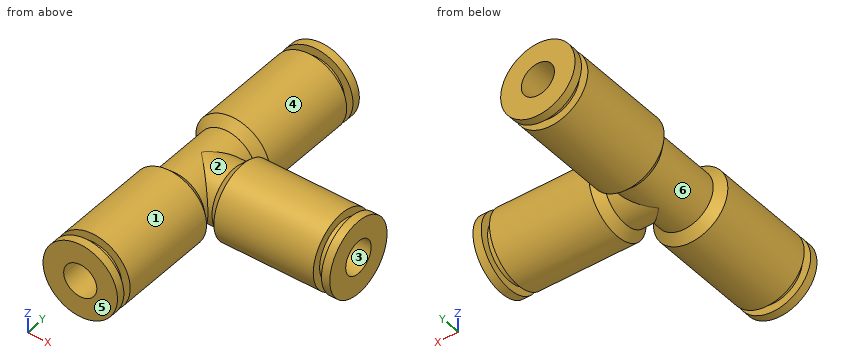
```python
from build123d import *
from build123d.topology import SkipClean

# Parameters (mm, degrees)
PATTERN_CIRCULAR_1_COUNT = 3
PATTERN_CIRCULAR_1_ANGLE = 180


with BuildPart() as part:
    # Эскиз1 one side → Повернуть1 (revolve)
    with BuildSketch(Plane.XY, mode=Mode.PRIVATE) as revolve_1_sk:
        with BuildLine():
            Line((0, -3.5), (0, -2))
            ThreePointArc((0, -2), (-1.414213562, -1.414213562), (-2, 0))
            Line((-2, 0), (-2, 6))
            Line((-2, 6), (-2, 19))
            Line((-2, 19), (-4.5, 19))
            Line((-4.5, 19), (-4.5, 18))
            Line((-4.5, 18), (-3.5, 18))
            Line((-3.5, 18), (-3.5, 17))
            Line((-3.5, 17), (-4.5, 17))
            Line((-4.5, 17), (-4.5, 5))
            Line((-4.5, 5), (-3.5, 4))
            Line((-3.5, 4), (-3.5, 0))
            ThreePointArc((-3.5, 0), (-2.474873734, -2.474873734), (0, -3.5))
        make_face()
    revolve_1 = revolve(revolve_1_sk.sketch.rotate(Axis((0, 0.887308405, 0), (0, 1, 0)), 180), axis=Axis((0, 0.887308405, 0), (0, 1, 0)))

    # Круговой массив1: Повернуть1 ×3 about axis
    with SkipClean():  # the faces are left unmerged after this step: merging them gives an invalid solid
        pattern_circular_1_axis = Axis((0, 0, 0), (0, 0, -1))
        for i in range(1, PATTERN_CIRCULAR_1_COUNT):
            add(revolve_1.rotate(pattern_circular_1_axis, i * PATTERN_CIRCULAR_1_ANGLE / (PATTERN_CIRCULAR_1_COUNT - 1)))


solid = part.part
```
Input: part model. Units: mm. Frame: model coordinates. Face numbers are marked on the shaded views. A direction names the side the tool comes from. Round coordinates to 2 decimals unless told otherwise and drop trailing zeros. Loops run counter-clockwise (first coordinate to the right, second up) from the corner with the lowest first, then second, coordinate; pieces in that order, holes last. Notation, with made-up numbers: M 85,43.25 L 92,43.25 A21 ccw 92,48.25 Z; hole C -39.5,56 d3. An arc over 180 degrees is marked long. Answer in a Markdown table with one row per item. Add a question column.
1. Section A-A (x = 14.75). Output: boundary loops of the cut face in (y, z).
2. Ray query, probe 1 along Z at (x, y) = (0, 9.5); probe 2 along X at (y, z) = (-3.5, -0.5); probe 3 along Y at (x, z) = (-3.25, 2). Return the intervals inside material, ascending.
3. Contact query for flat-ended pins moving along their axis: pin 1 (4.5 mm diameter, centred on x = 0, z = 0, fed in from +Y); pin 2 (2 mm diameter, centred on x = 4.5, y = 5.5, fed in from -Z); pin 3 (3.5 mm diameter, centred on x = 0, z = 0, fed in from +Y); pin 4 (1.5 mm diameter, centred on x = 6.5, z = -1, fed in from -Y). Output: stop coordinate, or through.
4. Mould query, pull axis Y, two halves, no side actions, for the marked faces 4, 5 and 6. Classes: released by +Y, released by -Y, zero draft, split by the parting line, or undercut.
5. Set-up query: the marked faces 1, 2 and 3. Return all of +Z, -Z, +X, -X, +Y, -Y with unobstructed straight access to the full face (end or side cutting, diameter ignored); none if empty.
Values follow:
| question | item | result |
|---|---|---|
| 1 | outline | C 0,0 d9; hole C 0,0 d4 |
| 2 | probe 1 | -4.5 to -2, 2 to 4.5 |
| 2 | probe 2 | -3.46 to -1.94, 1.94 to 3.46, 4.04 to 17, 18 to 19 |
| 2 | probe 3 | -19 to -18, -17 to -4.32, 4.32 to 17, 18 to 19 |
| 3 | pin 1 | y = 19 |
| 3 | pin 2 | z = -2.83 |
| 3 | pin 3 | y = 3.5 |
| 3 | pin 4 | y = -4.49 |
| 4 | face 4 | zero draft |
| 4 | face 5 | released by -Y |
| 4 | face 6 | undercut |
| 5 | face 1 | -Y |
| 5 | face 2 | none |
| 5 | face 3 | +X |
